from build123d import *

# Parameters (mm, degrees)
SKETCH_1_R      = 3.4
SKETCH_1_W      = 10.3
SKETCH_1_H      = 10.3
EXTRUDE_1_DEPTH = 100


with BuildPart() as part:
    # 草图1 → 凸台-拉伸1 (new body)
    with BuildSketch(Plane.XY):
        with BuildLine():
            Line((-4.582808051, 8.751402525), (-7.482808051, 8.751402525))
            Line((-7.482808051, 8.751402525), (-7.482808051, 17.151402525))
            Line((-7.482808051, 17.151402525), (-5.082808051, 17.151402525))
            ThreePointArc((-5.082808051, 17.151402525), (-4.72925466, 17.297849134), (-4.582808051, 17.651402525))
            Line((-4.582808051, 17.651402525), (-4.582808051, 19.651402525))
            ThreePointArc((-4.582808051, 19.651402525), (-4.72925466, 20.004955915), (-5.082808051, 20.151402525))
            Line((-5.082808051, 20.151402525), (-19.982808051, 20.151402525))
            ThreePointArc((-19.982808051, 20.151402525), (-20.336361441, 20.004955915), (-20.482808051, 19.651402525))
            Line((-20.482808051, 19.651402525), (-20.482808051, 4.751402525))
            ThreePointArc((-20.482808051, 4.751402525), (-20.336361441, 4.397849134), (-19.982808051, 4.251402525))
            Line((-19.982808051, 4.251402525), (-17.982808051, 4.251402525))
            ThreePointArc((-17.982808051, 4.251402525), (-17.62925466, 4.397849134), (-17.482808051, 4.751402525))
            Line((-17.482808051, 4.751402525), (-17.482808051, 7.151402525))
            Line((-17.482808051, 7.151402525), (-9.082808051, 7.151402525))
            Line((-9.082808051, 7.151402525), (-9.082808051, 4.251402525))
            Line((-9.082808051, 4.251402525), (-7.539914832, 5.794295743))
            Line((-7.539914832, 5.794295743), (-5.337353801, 3.591734712))
            ThreePointArc((-5.337353801, 3.591734712), (-6.432808051, 0.151402525), (-5.337353801, -3.288929663))
            Line((-5.337353801, -3.288929663), (-7.539914832, -5.491490694))
            Line((-7.539914832, -5.491490694), (-9.082808051, -3.948597475))
            Line((-9.082808051, -3.948597475), (-9.082808051, -6.848597475))
            Line((-9.082808051, -6.848597475), (-17.482808051, -6.848597475))
            Line((-17.482808051, -6.848597475), (-17.482808051, -4.448597475))
            ThreePointArc((-17.482808051, -4.448597475), (-17.62925466, -4.095044085), (-17.982808051, -3.948597475))
            Line((-17.982808051, -3.948597475), (-19.982808051, -3.948597475))
            ThreePointArc((-19.982808051, -3.948597475), (-20.336361441, -4.095044085), (-20.482808051, -4.448597475))
            Line((-20.482808051, -4.448597475), (-20.482808051, -19.348597475))
            ThreePointArc((-20.482808051, -19.348597475), (-20.336361441, -19.702150866), (-19.982808051, -19.848597475))
            Line((-19.982808051, -19.848597475), (-5.082808051, -19.848597475))
            ThreePointArc((-5.082808051, -19.848597475), (-4.72925466, -19.702150866), (-4.582808051, -19.348597475))
            Line((-4.582808051, -19.348597475), (-4.582808051, -17.348597475))
            ThreePointArc((-4.582808051, -17.348597475), (-4.72925466, -16.995044085), (-5.082808051, -16.848597475))
            Line((-5.082808051, -16.848597475), (-7.482808051, -16.848597475))
            Line((-7.482808051, -16.848597475), (-7.482808051, -8.448597475))
            Line((-7.482808051, -8.448597475), (-4.582808051, -8.448597475))
            Line((-4.582808051, -8.448597475), (-6.125701269, -6.905704257))
            Line((-6.125701269, -6.905704257), (-3.923140238, -4.703143225))
            ThreePointArc((-3.923140238, -4.703143225), (-0.482808051, -5.798597475), (2.957524137, -4.703143225))
            Line((2.957524137, -4.703143225), (5.160085168, -6.905704257))
            Line((5.160085168, -6.905704257), (3.617191949, -8.448597475))
            Line((3.617191949, -8.448597475), (6.517191949, -8.448597475))
            Line((6.517191949, -8.448597475), (6.517191949, -16.848597475))
            Line((6.517191949, -16.848597475), (4.117191949, -16.848597475))
            ThreePointArc((4.117191949, -16.848597475), (3.763638559, -16.995044085), (3.617191949, -17.348597475))
            Line((3.617191949, -17.348597475), (3.617191949, -19.348597475))
            ThreePointArc((3.617191949, -19.348597475), (3.763638559, -19.702150866), (4.117191949, -19.848597475))
            Line((4.117191949, -19.848597475), (19.017191949, -19.848597475))
            ThreePointArc((19.017191949, -19.848597475), (19.37074534, -19.702150866), (19.517191949, -19.348597475))
            Line((19.517191949, -19.348597475), (19.517191949, -4.448597475))
            ThreePointArc((19.517191949, -4.448597475), (19.37074534, -4.095044085), (19.017191949, -3.948597475))
            Line((19.017191949, -3.948597475), (17.017191949, -3.948597475))
            ThreePointArc((17.017191949, -3.948597475), (16.663638559, -4.095044085), (16.517191949, -4.448597475))
            Line((16.517191949, -4.448597475), (16.517191949, -6.848597475))
            Line((16.517191949, -6.848597475), (8.117191949, -6.848597475))
            Line((8.117191949, -6.848597475), (8.117191949, -3.948597475))
            Line((8.117191949, -3.948597475), (6.574298731, -5.491490694))
            Line((6.574298731, -5.491490694), (4.371737699, -3.288929663))
            ThreePointArc((4.371737699, -3.288929663), (5.467191949, 0.151402525), (4.371737699, 3.591734712))
            Line((4.371737699, 3.591734712), (6.574298731, 5.794295743))
            Line((6.574298731, 5.794295743), (8.117191949, 4.251402525))
            Line((8.117191949, 4.251402525), (8.117191949, 7.151402525))
            Line((8.117191949, 7.151402525), (16.517191949, 7.151402525))
            Line((16.517191949, 7.151402525), (16.517191949, 4.751402525))
            ThreePointArc((16.517191949, 4.751402525), (16.663638559, 4.397849134), (17.017191949, 4.251402525))
            Line((17.017191949, 4.251402525), (19.017191949, 4.251402525))
            ThreePointArc((19.017191949, 4.251402525), (19.37074534, 4.397849134), (19.517191949, 4.751402525))
            Line((19.517191949, 4.751402525), (19.517191949, 19.651402525))
            ThreePointArc((19.517191949, 19.651402525), (19.37074534, 20.004955915), (19.017191949, 20.151402525))
            Line((19.017191949, 20.151402525), (4.117191949, 20.151402525))
            ThreePointArc((4.117191949, 20.151402525), (3.763638559, 20.004955915), (3.617191949, 19.651402525))
            Line((3.617191949, 19.651402525), (3.617191949, 17.651402525))
            ThreePointArc((3.617191949, 17.651402525), (3.763638559, 17.297849134), (4.117191949, 17.151402525))
            Line((4.117191949, 17.151402525), (6.517191949, 17.151402525))
            Line((6.517191949, 17.151402525), (6.517191949, 8.751402525))
            Line((6.517191949, 8.751402525), (3.617191949, 8.751402525))
            Line((3.617191949, 8.751402525), (5.160085168, 7.208509306))
            Line((5.160085168, 7.208509306), (2.957524137, 5.005948275))
            ThreePointArc((2.957524137, 5.005948275), (-0.482808051, 6.101402525), (-3.923140238, 5.005948275))
            Line((-3.923140238, 5.005948275), (-6.125701269, 7.208509306))
            Line((-6.125701269, 7.208509306), (-4.582808051, 8.751402525))
        make_face()
        with Locations((-0.482808051, 0.151402525)):
            Circle(SKETCH_1_R, mode=Mode.SUBTRACT)
        with Locations((-13.632808051, 13.301402525)):
            Rectangle(SKETCH_1_W, SKETCH_1_H, mode=Mode.SUBTRACT)
        with Locations((12.667191949, 13.301402525)):
            Rectangle(SKETCH_1_W, SKETCH_1_H, mode=Mode.SUBTRACT)
        with Locations((-13.632808051, -12.998597475)):
            Rectangle(SKETCH_1_W, SKETCH_1_H, mode=Mode.SUBTRACT)
        with Locations((12.667191949, -12.998597475)):
            Rectangle(SKETCH_1_W, SKETCH_1_H, mode=Mode.SUBTRACT)
    extrude(amount=EXTRUDE_1_DEPTH)


solid = part.part
The listing builds one solid part. Answer for the finished solid, in the listing's coordinates (mm). A direction names the side the tool comes from. Give positions to 0.01 mm unless a question says otherwise; leave off trailing zeros. Loops run counter-clockwise (first coordinate to the right, second up) from the corner with the lowest first, then second, coordinate; pieces in that order, holes last. Notation, with made-up numbers: (46.5, 37.5) - (84.5, 37.5) arc R5 ccw to (84.5, 45.5) - close; hole circle Ø8 at (60.5, 30). An arc over 180 degrees is marked (long way). Answer as a JSON object with one key per item and string values.
1. A cutting plane is placed at A-A (x = -16). Write down the section's boundary in (y, z), then the cut area to 3 significant figures.
Determined:
{"outline": "(-19.85, 0) - (-18.15, 0) - (-18.15, 100) - (-19.85, 100) - close; (-7.85, 0) - (-6.85, 0) - (-6.85, 100) - (-7.85, 100) - close; (7.15, 0) - (8.15, 0) - (8.15, 100) - (7.15, 100) - close; (18.45, 0) - (20.15, 0) - (20.15, 100) - (18.45, 100) - close", "area": "540 mm²"}
2. A cutting plane is placed at B-B (y = 10.5). Write down the section's boundary in (x, z), then the cut area to 3 significant figures.
Determined:
{"outline": "(-20.48, 0) - (-18.78, 0) - (-18.78, 100) - (-20.48, 100) - close; (-8.48, 0) - (-7.48, 0) - (-7.48, 100) - (-8.48, 100) - close; (6.52, 0) - (7.52, 0) - (7.52, 100) - (6.52, 100) - close; (17.82, 0) - (19.52, 0) - (19.52, 100) - (17.82, 100) - close", "area": "540 mm²"}
3. Find the intervals of material crossed by L1, parallel to Y at x = -17, z = 59; L2, parallel to X at y = 12, z = 26; L3, parallel to Y at x = 8, z = 64, in increasing order. Write a range as [from, to].
Determined:
{"L1": "[-19.85, -18.15], [-7.85, -6.85], [7.15, 8.15], [18.45, 20.15]", "L2": "[-20.48, -18.78], [-8.48, -7.48], [6.52, 7.52], [17.82, 19.52]", "L3": "[-19.85, -18.15], [-7.85, -4.07], [4.37, 8.15], [18.45, 20.15]"}
4. For faces 4 (the flat face through (3.617, -18, 49)), 5 (the flat face through (19.517, 12, 49)), 6 (the flat face through (5, 8.751, 49)), determine the directions among +Z, -Z, +X, -X, +Y, -Y from which every point of the face is accessible in a straight line to the end or side of a thin tool.
Determined:
{"face 4": "+Z, -Z, -Y", "face 5": "+Z, -Z, +X, +Y, -Y", "face 6": "+Z, -Z"}
5. For a pull along Y with two mould halves and no side action, classify faces 1 (the flat face through (-12, 20.151, 49)), 2 (the flat face through (-4, 2, 100)), 3 (the flat face through (7.517, -13, 49)) as pulls with the +Y half, pulls with the -Y half, needs draft (parallel to the pull), parting line crosses it, or undercut.
Determined:
{"face 1": "pulls with the +Y half", "face 2": "needs draft", "face 3": "undercut"}
6. A cutting plane is placed at D-D (y = 2). Write down the section's boundary in (x, z).
Determined:
{"outline": "(-6.14, 0) - (-3.34, 0) - (-3.34, 100) - (-6.14, 100) - close; (2.37, 0) - (5.17, 0) - (5.17, 100) - (2.37, 100) - close"}
7. A cutting plane is placed at C-C (x = -0.5). Write down the section's boundary in (y, z).
Determined:
{"outline": "(-5.8, 0) - (-3.25, 0) - (-3.25, 100) - (-5.8, 100) - close; (3.55, 0) - (6.1, 0) - (6.1, 100) - (3.55, 100) - close"}
